from build123d import *


with BuildPart() as part:
    # Sketch2 → Revolve1 (revolve)
    with BuildSketch(Plane.XY, mode=Mode.PRIVATE) as revolve1_sk:
        with BuildLine():
            Line((20.955, 30.48), (20.955, 12.7))
            Line((20.955, 12.7), (22.225, 12.7))
            Line((22.225, 12.7), (22.225, 0))
            Line((22.225, 0), (28.575, 0))
            Line((28.575, 0), (28.575, 1.5875))
            Line((28.575, 1.5875), (25.4, 1.5875))
            Line((25.4, 1.5875), (25.4, 11.1125))
            Line((25.4, 11.1125), (28.575, 11.1125))
            Line((28.575, 11.1125), (28.575, 12.7))
            Line((28.575, 12.7), (26.67, 12.7))
            Line((26.67, 12.7), (26.67, 15.079229731))
            Line((26.67, 15.079229731), (23.368, 15.079229731))
            Line((23.368, 15.079229731), (23.368, 30.48))
            ThreePointArc((23.368, 30.48), (26.699072346, 40.209619932), (35.294362711, 45.856081704))
            ThreePointArc((35.294362711, 45.856081704), (36.355227336, 47.693893747), (34.495528336, 48.715904748))
            ThreePointArc((34.495528336, 48.715904748), (24.710263402, 41.836651461), (20.955, 30.48))
        make_face()
    revolve(revolve1_sk.sketch.rotate(Axis((0, 0, 0), (0, 1, 0)), 90), axis=Axis((0, 0, 0), (0, 1, 0)))


solid = part.part
Geometry check sheet. Reference: the model listing, model coordinates, mm. A direction names the side the tool comes from. Round coordinates to 2 decimals unless told otherwise and drop trailing zeros. Write each loop counter-clockwise with the first axis right and the second up, starting at its lowest first coordinate (ties: lowest second). Pieces come first, ordered by that corner, then holes. Notation, with made-up numbers: (-7, 35.25) - (48, 35.25) arc R19 cw to (48, 45.25) - close; hole circle Ø11 at (-32, 25.5). An arc over 180 degrees is marked (long way). One line per item, written item: value.
1. Mould release check, pull along Y, two halves, no side actions. Record for faces 1 (the face through (2, 1.588, 26)), 2 (the face through (19, 12.7, -19)), 3 (the face through (17, 0, 15)), 4 (the face through (-20.777, 21.466, 2.728)): released by +Y, released by -Y, zero draft, split by the parting line, or undercut.
The answers:
face 1: undercut
face 2: undercut
face 3: released by -Y
face 4: zero draft
2. Depth check by flat-ended pin: pin 1 Ø1.5 at (x, y) = (-18, 24) entering from -Z; pin 2 Ø3 at (y, z) = (39, 23.5) entering from -X; pin 3 Ø10 at (y, z) = (23.5, -1) entering from -X; pin 4 Ø17 at (x, z) = (-2, -11.5) entering from -Y. Enter the tip coordinate at first touch or a pass-through.
The answers:
pin 1: stops at z = -15.76
pin 2: stops at x = -14.26
pin 3: stops at x = -23.37
pin 4: passes through
3. Cross-section at C-C on y = 26. Record the boundary of the cut face in (x, z) (3 decimals), and give its area (3 significant figures).
The answers:
outline: circle Ø46.736 at (0, 0); hole circle Ø41.91 at (0, 0)
area: 336 mm^2
4. Set-up check for faces 5 (the face through (-7, 12.7, -20)), 6 (the face through (24, 15.079, 0)): record each of +Z, -Z, +X, -X, +Y, -Y from which the full face is reachable in a straight line by a thin tool's end or side.
The answers:
face 5: -Y
face 6: none
5. Scan lines: L1, parallel to X at y = 25, z = 0 (3 decimals); L2, parallel to X at y = 8, z = 0 (3 decimals); L3, parallel to Y at x = 25.5, z = -2. Record each from-to range of solid material in increasing order.
The answers:
L1: x = -23.368 to -20.955, 20.955 to 23.368
L2: x = -25.4 to -22.225, 22.225 to 25.4
L3: y = 0 to 1.59, 11.11 to 15.08, 38.56 to 42.92
6. Cross-section at D-D on y = 9.5. Record the boundary of the cut face in (x, z) (3 decimals), and give its area (3 significant figures).
The answers:
outline: circle Ø50.8 at (0, 0); hole circle Ø44.45 at (0, 0)
area: 475 mm^2
